Could you check a few things on this model? Use its own coordinates, in mm. A direction names the side the tool comes from. Round coordinates to 2 decimals unless told otherwise and drop trailing zeros. Loops run counter-clockwise (first coordinate to the right, second up) from the corner with the lowest first, then second, coordinate; pieces in that order, holes last. Notation, with made-up numbers: (49, 8) -> (83, 8) arc R9 cw to (83, 22) -> close; hole circle Ø7 at (13, -21). An arc over 180 degrees is marked (long way). Write each question's results on one line, items separated by ' | '.
from build123d import *

# Parameters (mm, degrees)
SKETCH1_W           = 95.7
SKETCH1_H           = 100
SKETCH1_R           = 1.6
BOSS_EXTRUDE1_DEPTH = 3
SKETCH2_W           = 84.114636839
SKETCH2_H           = 30
SKETCH2_R           = 1.6
BOSS_EXTRUDE2_DEPTH = 5
SKETCH3_W           = 7
SKETCH3_H           = 30
BOSS_EXTRUDE3_DEPTH = 23
SKETCH4_R           = 1.6
CUT_EXTRUDE1_DEPTH  = 114
SKETCH5_W           = 95.7
SKETCH5_H           = 6
CUT_EXTRUDE2_DEPTH  = 114


with BuildPart() as part:
    # Sketch1 → Boss-Extrude1 (new body, symmetric)
    with BuildSketch(Plane(origin=(0, 0, 0), x_dir=(1, 0, 0), z_dir=(0, 1, 0))):
        Rectangle(SKETCH1_W, SKETCH1_H)
        with Locations((-8.75, 45.181367204)):
            Circle(SKETCH1_R, mode=Mode.SUBTRACT)
        with Locations((8.75, 45.181367204)):
            Circle(SKETCH1_R, mode=Mode.SUBTRACT)
        with Locations((0, -46)):
            Circle(SKETCH1_R, mode=Mode.SUBTRACT)
    extrude(amount=BOSS_EXTRUDE1_DEPTH, both=True)

    # Sketch2 → Boss-Extrude2 (add)
    with BuildSketch(Plane(origin=(0, 3, 0), x_dir=(1, 0, 0), z_dir=(0, 1, 0))):
        with Locations((0.497719744, 35)):
            Rectangle(SKETCH2_W, SKETCH2_H)
        with Locations((-8.75, 45.181367204)):
            Circle(SKETCH2_R, mode=Mode.SUBTRACT)
        with Locations((8.75, 45.181367204)):
            Circle(SKETCH2_R, mode=Mode.SUBTRACT)
        with Locations((0.497719744, 35)):
            Rectangle(SKETCH2_W, SKETCH2_H)
        with Locations((-8.75, 45.181367204)):
            Circle(SKETCH2_R, mode=Mode.SUBTRACT)
        with Locations((8.75, 45.181367204)):
            Circle(SKETCH2_R, mode=Mode.SUBTRACT)
    extrude(amount=BOSS_EXTRUDE2_DEPTH)

    # Sketch3 → Boss-Extrude3 (add)
    with BuildSketch(Plane(origin=(0, 8, 0), x_dir=(1, 0, 0), z_dir=(0, 1, 0))):
        with Locations((-38.059598675, 35)):
            Rectangle(SKETCH3_W, SKETCH3_H)
        with Locations((39.055038164, 35)):
            Rectangle(SKETCH3_W, SKETCH3_H)
    extrude(amount=BOSS_EXTRUDE3_DEPTH)

    # Sketch4 → Cut-Extrude1 (cut)
    with BuildSketch(Plane.ZY.offset(41.559598675)):
        with Locations((-29, 26.474830264)):
            Circle(SKETCH4_R)
    extrude(amount=-CUT_EXTRUDE1_DEPTH, mode=Mode.SUBTRACT)

    # Sketch5 → Cut-Extrude2 (cut)
    with BuildSketch(Plane.XY.offset(50)):
        Rectangle(SKETCH5_W, SKETCH5_H)
    extrude(amount=-CUT_EXTRUDE2_DEPTH, mode=Mode.SUBTRACT)


solid = part.part
1) For faces 4 (the cylindrical face through (-10.35, 5.46, -45.25)), 5 (the flat face through (35.555, 19, -35)), which set-ups out of +Z, -Z, +X, -X, +Y, -Y let a thin tool reach every point of the face, with its end or its side?
Model answer:
face 4: +Y, -Y | face 5: +Z, -Z, +Y
2) I want a section at B-B, the plane x = -8.75. Write out the boundary of the cut face in (y, z).
Model answer:
outline: (3, -50) -> (8, -50) -> (8, -46.78) -> (3, -46.78) -> close; (3, -43.58) -> (8, -43.58) -> (8, -20) -> (3, -20) -> close
3) If we mould it in two halves opening along Z, with no side actions, what happens to faces 1 (the cylindrical face through (7.15, 5.46, -45.25)), 2 (the flat face through (-41.56, 17, -35)), 3 (the flat face through (0, 7, -20))? For each: released by +Z, released by -Z, zero draft, split by the parting line, or undercut.
Model answer:
face 1: undercut | face 2: zero draft | face 3: released by +Z
4) I want a section at C-C, the plane z = -29. Write out the boundary of the cut face in (x, y).
Model answer:
outline: (-41.56, 3) -> (42.56, 3) -> (42.56, 24.87) -> (35.56, 24.87) -> (35.56, 8) -> (-34.56, 8) -> (-34.56, 24.87) -> (-41.56, 24.87) -> close; (-41.56, 28.07) -> (-34.56, 28.07) -> (-34.56, 31) -> (-41.56, 31) -> close; (35.56, 28.07) -> (42.56, 28.07) -> (42.56, 31) -> (35.56, 31) -> close
5) I want a section at D-D, the plane x = -30.5. Write out the boundary of the cut face in (y, z), plus the area to 3 significant figures.
Model answer:
outline: (3, -50) -> (8, -50) -> (8, -20) -> (3, -20) -> close | area: 150 mm2
6) I want a section at A-A, the plane y = 21.75. Write out the boundary of the cut face in (x, z).
Model answer:
outline: (-41.56, -50) -> (-34.56, -50) -> (-34.56, -20) -> (-41.56, -20) -> close; (35.56, -50) -> (42.56, -50) -> (42.56, -20) -> (35.56, -20) -> close
7) I need wall thicknesses on line 1 (X direction, y = 15.75, z = -25.5); line 2 (Y direction, x = 37, z = -29); line 3 (Z direction, x = 8.75, y = 4). Which ranges of each line are inside material? Lowest first, please.
Model answer:
line 1: x = -41.56 to -34.56, 35.56 to 42.56 | line 2: y = 3 to 24.87, 28.07 to 31 | line 3: z = -50 to -46.78, -43.58 to -20
